The model under review builds one solid part; all positions refer to its coordinate system, in mm. A direction names the side the tool comes from. Round coordinates to 2 decimals unless told otherwise and drop trailing zeros. Write each loop counter-clockwise with the first axis right and the second up, starting at its lowest first coordinate (ties: lowest second). Pieces come first, ordered by that corner, then holes. Notation, with made-up numbers: (16.25, 6.5) - (67.25, 6.5) arc R5 cw to (67.25, 10.5) - close; hole circle Ø9 at (-37.5, 73). An arc over 180 degrees is marked (long way). Use one line per item in the form item = value.
from build123d import *

# Parameters (mm, degrees)
CROQUIS1_R              = 2.05
CROQUIS1_R_2            = 1.5
SALIENTE_EXTRUIR1_DEPTH = 4.84


with BuildPart() as part:
    # Croquis1 → Saliente-Extruir1 (new body)
    with BuildSketch(Plane(origin=(0, 0, 0), x_dir=(0, 0, -1), z_dir=(1, 0, 0))):
        Polygon((-10, 0), (-10, 71.56), (-7.5, 71.56), (-7.5, 74), (7.5, 74), (7.5, 71.56), (10, 71.56), (10, -39.56), (7.5, -39.56), (7.5, -42), (-7.5, -42), (-7.5, -39.56), (-10, -39.56), align=None)
        with Locations((4.31, 0)):
            Circle(CROQUIS1_R, mode=Mode.SUBTRACT)
        with Locations((-4.5, 8.81)):
            Circle(CROQUIS1_R_2, mode=Mode.SUBTRACT)
        with Locations((-4.5, -8.81)):
            Circle(CROQUIS1_R_2, mode=Mode.SUBTRACT)
    extrude(amount=SALIENTE_EXTRUIR1_DEPTH)


solid = part.part
(1) Machinability: for faces 1 (the flat face through (2, 73, -7.5)), 2 (the flat face through (2, -41, 7.5)), 3 (the flat face through (2, 73, 7.5)), which of the approach directions +Z, -Z, +X, -X, +Y, -Y give a long, thin tool a straight path to every point of the face, cutting with its end or side? Answer none if there is none.
Geometry results:
face_1 = -Z, +X, -X, +Y
face_2 = +Z, +X, -X, -Y
face_3 = +Z, +X, -X, +Y
(2) To check wall thickness, follow L1, parallel to Y at x = 3.5, z = 4.5; L2, parallel to Y at x = 2, z = -4.31; L3, parallel to Y at x = 3.05, z = -3. State the ranges of each line that lie inside material, in increasing order.
Geometry results:
L1 = -42 to -10.31, -7.31 to 7.31, 10.31 to 74
L2 = -42 to -2.05, 2.05 to 74
L3 = -42 to -1.58, 1.58 to 74
(3) Add section D-D on z = 4.5. Write out the cut boundary in (x, y), then the cut area to 3 significant figures.
Geometry results:
outline = (0, -42) - (4.84, -42) - (4.84, -10.31) - (0, -10.31) - close; (0, -7.31) - (4.84, -7.31) - (4.84, 7.31) - (0, 7.31) - close; (0, 10.31) - (4.84, 10.31) - (4.84, 74) - (0, 74) - close
area = 532 mm2
(4) Add section C-C on x = 3.8. Write out the cut boundary in (y, z), then the cut area to 3 significant figures.
Geometry results:
outline = (-42, -7.5) - (-39.56, -7.5) - (-39.56, -10) - (71.56, -10) - (71.56, -7.5) - (74, -7.5) - (74, 7.5) - (71.56, 7.5) - (71.56, 10) - (-39.56, 10) - (-39.56, 7.5) - (-42, 7.5) - close; hole circle Ø3 at (-8.81, 4.5); hole circle Ø4.1 at (0, -4.31); hole circle Ø3 at (8.81, 4.5)
area = 2,270 mm2
(5) The part is to be moulded in two halves that separate along Z. For faces 4 (the flat face through (2, -41, -7.5)), 5 (the flat face through (2, 71.56, -9)), 6 (the cylindrical face through (2.39, 0.09, -2.26)), say which applies: +Z half, -Z half, draft (parallel to the pull), parting line (faces both ways), or undercut.
Geometry results:
face_4 = -Z half
face_5 = draft
face_6 = undercut
(6) Add section B-B on z = -4.31. Write out the cut boundary in (x, y), then the cut area to 3 significant figures.
Geometry results:
outline = (0, -42) - (4.84, -42) - (4.84, -2.05) - (0, -2.05) - close; (0, 2.05) - (4.84, 2.05) - (4.84, 74) - (0, 74) - close
area = 542 mm2
(7) Insertion check: P1, Ø2.5, axis at x = 3.5, y = -41, coming from the -Z side; P2, Ø2, axis at x = 2.5, y = 73.5, coming from the +Z side; P3, Ø0.8, axis at x = 3, z = 8.5, coming from the -Y side. Each pin has a flat end and moves straight along its axis. Give the tip position at first contact, or say it passes through.
Geometry results:
P1 = -7.5
P2 = 7.5
P3 = -39.56
(8) Add section A-A on y = 0. Write out the cut boundary in (x, z), then the cut area to 3 significant figures.
Geometry results:
outline = (0, -10) - (4.84, -10) - (4.84, -6.36) - (0, -6.36) - close; (0, -2.26) - (4.84, -2.26) - (4.84, 10) - (0, 10) - close
area = 77.0 mm2
